```python
from build123d import *

# Parameters (mm, degrees)
BASE_FLANGE1_DEPTH = 101.6
EDGE_FLANGE1_START = -94.5134
EDGE_FLANGE1_DEPTH = 189.0268


# Read off the part's stored shape, not the designer's step: Edge-Flange1
# Sheet-metal steps are written as plain solids
with BuildPart() as part:
    # Sketch1 → Base-Flange1 (new body)
    with BuildSketch(Plane(origin=(0, 0, 0), x_dir=(1, 0, 0), z_dir=(0, 1, 0))):
        with BuildLine():
            Line((-123.825, 0), (-99.1616, 0))
            ThreePointArc((-99.1616, 0), (-96.395681115, -1.145681115), (-95.25, -3.9116))
            Line((-95.25, -3.9116), (-95.25, -88.1634))
            ThreePointArc((-95.25, -88.1634), (-95.034254855, -88.684254855), (-94.5134, -88.9))
            Line((-94.5134, -88.9), (94.5134, -88.9))
            ThreePointArc((94.5134, -88.9), (95.034254855, -88.684254855), (95.25, -88.1634))
            Line((95.25, -88.1634), (95.25, -3.9116))
            ThreePointArc((95.25, -3.9116), (96.395681115, -1.145681115), (99.1616, 0))
            Line((99.1616, 0), (123.825, 0))
            Line((123.825, 0), (123.825, -3.175))
            Line((123.825, -3.175), (99.1616, -3.175))
            ThreePointArc((99.1616, -3.175), (98.640745145, -3.390745145), (98.425, -3.9116))
            Line((98.425, -3.9116), (98.425, -88.1634))
            ThreePointArc((98.425, -88.1634), (97.279318885, -90.929318885), (94.5134, -92.075))
            Line((94.5134, -92.075), (-94.5134, -92.075))
            ThreePointArc((-94.5134, -92.075), (-97.279318885, -90.929318885), (-98.425, -88.1634))
            Line((-98.425, -88.1634), (-98.425, -3.9116))
            ThreePointArc((-98.425, -3.9116), (-98.640745145, -3.390745145), (-99.1616, -3.175))
            Line((-99.1616, -3.175), (-123.825, -3.175))
            Line((-123.825, -3.175), (-123.825, 0))
        make_face()
    extrude(amount=BASE_FLANGE1_DEPTH)

    # Edge-Flange1 outline → Edge-Flange1 (add)
    with BuildSketch(Plane.YZ.offset(EDGE_FLANGE1_START)):
        with BuildLine():
            Line((-69.85, 0), (-66.675, 0))
            Line((-66.675, 0), (-66.675, 88.1634))
            ThreePointArc((-66.675, 88.1634), (-66.459254855, 88.684254855), (-65.9384, 88.9))
            Line((-65.9384, 88.9), (0, 88.9))
            Line((0, 88.9), (0, 92.075))
            Line((0, 92.075), (-65.9384, 92.075))
            ThreePointArc((-65.9384, 92.075), (-68.704318885, 90.929318885), (-69.85, 88.1634))
            Line((-69.85, 88.1634), (-69.85, 0))
        make_face()
    extrude(amount=EDGE_FLANGE1_DEPTH)


solid = part.part
```
The listing builds one solid part. Answer for the finished solid, in the listing's coordinates (mm). A direction names the side the tool comes from. Coordinates: 2 decimals unless noted, no trailing zeros. Write each loop counter-clockwise with the first axis right and the second up, starting at its lowest first coordinate (ties: lowest second). Pieces come first, ordered by that corner, then holes.
Q1. Find the intervals of material crossed by line 1 along X through (y, z) = (72.5, 47) (3 decimals); line 2 along Y through (x, z) = (31, 81.5) (3 decimals); line 3 along Z through (x, y) = (18, -22) (3 decimals), in increasing order.
Returned:
line 1: x = -98.425 to -95.25, 95.25 to 98.425
line 2: y = -69.85 to -66.675
line 3: z = 88.9 to 92.075
Q2. Given P1, Ø4, axis at x = -95.5, y = 79, coming from the +Z side (3 decimals); P2, Ø12.5, axis at x = -107.5, y = 49.5, coming from the +Z side (3 decimals); P3, Ø8, axis at x = -27, z = 77.5, coming from the +Y side (3 decimals); P4, Ø1.5, axis at x = -39, y = -10.5, coming from the -Z side, each flat-ended and moving along its own axis, determine where each tip first touches the part or whether it passes through.
Returned:
P1: stops at z = 92.075
P2: stops at z = 3.175
P3: stops at y = -66.675
P4: stops at z = 88.9
Q3. Section D-D, the plane y = -16 is taken. Write down the section's boundary in (x, z) (3 decimals).
Returned:
outline: (-94.513, 88.9) - (94.513, 88.9) - (94.513, 92.075) - (-94.513, 92.075) - close
Q4. Section B-B, the plane x = 65 is taken. Write down the section's boundary in (y, z) (3 decimals), then the cut area to 3 significant figures.
Returned:
outline: (-69.85, 0) - (-66.675, 0) - (-66.675, 88.163) arc R0.737 cw to (-65.938, 88.9) - (101.6, 88.9) - (101.6, 92.075) - (-65.938, 92.075) arc R3.912 ccw to (-69.85, 88.163) - close
area: 823 mm2
Q5. Section A-A, the plane z = 41.5 is taken. Write down the section's boundary in (x, y) (3 decimals), then the cut area to 3 significant figures.
Returned:
outline: (-98.425, 0) - (-95.25, 0) - (-95.25, 101.6) - (-98.425, 101.6) - close; (-94.513, -69.85) - (94.513, -69.85) - (94.513, -66.675) - (-94.513, -66.675) - close; (95.25, 0) - (98.425, 0) - (98.425, 101.6) - (95.25, 101.6) - close
area: 1,250 mm2
Q6. Section C-C, the plane y = 31 is taken. Write down the section's boundary in (x, z) (3 decimals).
Returned:
outline: (-123.825, 0) - (-99.162, 0) arc R3.912 ccw to (-95.25, 3.912) - (-95.25, 88.163) arc R0.737 cw to (-94.513, 88.9) - (94.513, 88.9) arc R0.737 cw to (95.25, 88.163) - (95.25, 3.912) arc R3.912 ccw to (99.162, 0) - (123.825, 0) - (123.825, 3.175) - (99.162, 3.175) arc R0.737 cw to (98.425, 3.912) - (98.425, 88.163) arc R3.912 ccw to (94.513, 92.075) - (-94.513, 92.075) arc R3.912 ccw to (-98.425, 88.163) - (-98.425, 3.912) arc R0.737 cw to (-99.162, 3.175) - (-123.825, 3.175) - close
Q7. Which of the six approach directions +Z, -Z, +X, -X, +Y, -Y give full straight-line access (tool end or side, diameter ignored) to faces 1 (the flat face through (-111, 50, 3.175)), 2 (the flat face through (112, 50, 3.175)), 3 (the flat face through (94.513, -69, 67))?
Returned:
face 1: +Z, -X, +Y, -Y
face 2: +Z, +X, +Y, -Y
face 3: +Z, -Z, +X, -Y
